```python
from build123d import *

# Parameters (mm, degrees)
ESTRUSIONE_ESTRUSIONE1_DEPTH = 17
TAGLIO_ESTRUSIONE1_DEPTH     = 321.60723635
RACCORDO1_R                  = 5
SCHIZZO3_R                   = 3
TAGLIO_ESTRUSIONE2_DEPTH     = 318.350542139
SCHIZZO4_W                   = 10
SCHIZZO4_H                   = 80
TAGLIO_ESTRUSIONE4_DEPTH     = 318.350542139
SCHIZZO5_R                   = 3
TAGLIO_ESTRUSIONE5_DEPTH     = 318.350542139


with BuildPart() as part:
    # Schizzo1 → Estrusione-Estrusione1 (new body)
    with BuildSketch(Plane.XY):
        with BuildLine():
            Line((160, 150), (200, 150))
            ThreePointArc((200, 150), (0, 250), (-200, 150))
            Line((-200, 150), (-160, 150))
            Line((-160, 150), (-160, -150))
            Line((-160, -150), (-200, -150))
            ThreePointArc((-200, -150), (0, -250), (200, -150))
            Line((200, -150), (160, -150))
            Line((160, -150), (160, 150))
        make_face()
    extrude(amount=ESTRUSIONE_ESTRUSIONE1_DEPTH)

    # Schizzo2 → Taglio-Estrusione1 (cut, through all)
    with BuildSketch(Plane.XY.offset(17)):
        with BuildLine():
            Line((-140, 33.25), (-100, 33.25))
            ThreePointArc((-100, 33.25), (-96.75, 30), (-100, 26.75))
            Line((-100, 26.75), (-140, 26.75))
            ThreePointArc((-140, 26.75), (-143.25, 30), (-140, 33.25))
        make_face()
        with BuildLine():
            Line((-140, -33.25), (-100, -33.25))
            ThreePointArc((-100, -33.25), (-96.75, -30), (-100, -26.75))
            Line((-100, -26.75), (-140, -26.75))
            ThreePointArc((-140, -26.75), (-143.25, -30), (-140, -33.25))
        make_face()
        with BuildLine():
            Line((140, -33.25), (100, -33.25))
            ThreePointArc((100, -33.25), (96.75, -30), (100, -26.75))
            Line((100, -26.75), (140, -26.75))
            ThreePointArc((140, -26.75), (143.25, -30), (140, -33.25))
        make_face()
        with BuildLine():
            Line((140, 33.25), (100, 33.25))
            ThreePointArc((100, 33.25), (96.75, 30), (100, 26.75))
            Line((100, 26.75), (140, 26.75))
            ThreePointArc((140, 26.75), (143.25, 30), (140, 33.25))
        make_face()
    extrude(amount=-TAGLIO_ESTRUSIONE1_DEPTH, mode=Mode.SUBTRACT)

    # Raccordo1
    raccordo1_edges = [part.edges().sort_by_distance(p)[0] for p in [
        (160, 150, 8.5),
        (160, -150, 8.5),
        (200, -150, 8.5),
        (-200, -150, 8.5),
        (-160, -150, 8.5),
        (-160, 150, 8.5),
        (-200, 150, 8.5),
        (200, 150, 8.5),
    ]]
    fillet(raccordo1_edges, radius=RACCORDO1_R)

    # Schizzo3 → Taglio-Estrusione2 (cut, through all)
    with BuildSketch(Plane(origin=(0, 0, 0), x_dir=(-1, 0, 0), z_dir=(0, 0, -1))):
        with Locations((-25, 180)):
            Circle(SCHIZZO3_R)
        with Locations(Location((25, 180, 0), (0, 0, 180))):
            Circle(SCHIZZO3_R)
        with Locations((-25, 105)):
            Circle(SCHIZZO3_R)
        with Locations((25, 105)):
            Circle(SCHIZZO3_R)
        with Locations(Location((-25, -105, 0), (0, 0, 180))):
            Circle(SCHIZZO3_R)
        with Locations(Location((25, -105, 0), (0, 0, 180))):
            Circle(SCHIZZO3_R)
        with Locations((25, -180)):
            Circle(SCHIZZO3_R)
        with Locations(Location((-25, -180, 0), (0, 0, 180))):
            Circle(SCHIZZO3_R)
    extrude(amount=-TAGLIO_ESTRUSIONE2_DEPTH, mode=Mode.SUBTRACT)

    # Schizzo4 → Taglio-Estrusione4 (cut, through all)
    with BuildSketch(Plane(origin=(0, 0, 0), x_dir=(-1, 0, 0), z_dir=(0, 0, -1))):
        with Locations((-60, 0)):
            Rectangle(SCHIZZO4_W, SCHIZZO4_H)
        with Locations((60, 0)):
            Rectangle(SCHIZZO4_W, SCHIZZO4_H)
    extrude(amount=-TAGLIO_ESTRUSIONE4_DEPTH, mode=Mode.SUBTRACT)

    # Schizzo5 → Taglio-Estrusione5 (cut, through all)
    with BuildSketch(Plane(origin=(0, 0, 0), x_dir=(-1, 0, 0), z_dir=(0, 0, -1))):
        with Locations((-170, 165)):
            Circle(SCHIZZO5_R)
        with Locations(Location((170, 165, 0), (0, 0, 180))):
            Circle(SCHIZZO5_R)
        with Locations((170, -165)):
            Circle(SCHIZZO5_R)
        with Locations(Location((-170, -165, 0), (0, 0, 180))):
            Circle(SCHIZZO5_R)
    extrude(amount=-TAGLIO_ESTRUSIONE5_DEPTH, mode=Mode.SUBTRACT)


solid = part.part
```
Build history of the part. All positions in model axes, mm. A direction names the side the tool comes from. Round coordinates to 2 decimals unless told otherwise and drop trailing zeros. Order: outer loops, then holes, each group sorted by start corner. A loop starts at its lowest first (then second) coordinate and runs counter-clockwise, first axis right, second up. Notation, with made-up numbers: (-36.75, 47.25) - (-0.75, 47.25) arc R14 cw to (-0.75, 64.25) - close; hole circle Ø2 at (36, 6.25). An arc over 180 degrees is marked (long way). Use a Markdown table: item, result.
1) Flat gauge pins, fed straight in: pin 1 Ø5 at (x, z) = (123, 11.5) entering from -Y; pin 2 Ø3 at (x, z) = (-61, 11) entering from -Y; pin 3 Ø5.5 at (x, y) = (170, -165) entering from -Z; pin 4 Ø5 at (y, z) = (-37.5, 9.5) entering from +X. Where does each tip first touch, or does it go through?
Recorded:
| item | result |
|---|---|
| pin 1 | stops at y = -219.04 |
| pin 2 | stops at y = -242.82 |
| pin 3 | passes through |
| pin 4 | stops at x = 160 |
2) Saw through at C-C on y = 126.5. Write the cut outline in (x, z), and give its area (3 significant figures).
Recorded:
| item | result |
|---|---|
| outline | (-160, 0) - (160, 0) - (160, 17) - (-160, 17) - close |
| area | 5,440 mm² |
3) Saw through at B-B on z = 12. Give the number of separate pieces and of enclosed holes in the cut face, and give its area (3 significant figures).
Recorded:
| item | result |
|---|---|
| separate pieces | 1 |
| enclosed holes | 18 |
| area | 149,000 mm² |
4) Wall check: L1, parallel to X at y = 38, z = 6.5; L2, parallel to Y at x = 172, z = 7.25; L3, parallel to Y at x = 130, z = 3.75. Give the ranges that are in metal, low to high.
Recorded:
| item | result |
|---|---|
| L1 | x = -160 to -65, -55 to 55, 65 to 160 |
| L2 | y = -181.43 to -167.24, -162.76 to -150, 150 to 162.76, 167.24 to 181.43 |
| L3 | y = -213.54 to -33.25, -26.75 to 26.75, 33.25 to 213.54 |
5) Tool access for faces 4 (the face through (177, 150, 8)), 5 (the face through (-3, 4, 0)), 6 (the face through (-120, 26.75, 9)), 7 (the face through (-160, 2, 8)): list every direction of +Z, -Z, +X, -X, +Y, -Y with a clear straight run to the whole face (end or side of a thin tool).
Recorded:
| item | result |
|---|---|
| face 4 | +Z, -Z, +X |
| face 5 | -Z, +X, -X, +Y, -Y |
| face 6 | +Z, -Z |
| face 7 | +Z, -Z, -X |
6) Saw through at A-A on x = 122. Write the cut outline in (y, z), and give its area (3 significant figures).
Recorded:
| item | result |
|---|---|
| outline | (-218.21, 0) - (-33.25, 0) - (-33.25, 17) - (-218.21, 17) - close; (-26.75, 0) - (26.75, 0) - (26.75, 17) - (-26.75, 17) - close; (33.25, 0) - (218.21, 0) - (218.21, 17) - (33.25, 17) - close |
| area | 7,200 mm² |
7) Pull direction Y, two halves, no side cores. Call faces 1 (the face through (3.1, 249.98, 8.38)), 2 (the face through (-120, -33.25, 9)), 3 (the face through (-3, 4, 17)): pulls with the +Y half, pulls with the -Y half, needs draft (parallel to the pull), parting line crosses it, or undercut.
Recorded:
| item | result |
|---|---|
| face 1 | pulls with the +Y half |
| face 2 | undercut |
| face 3 | needs draft |
